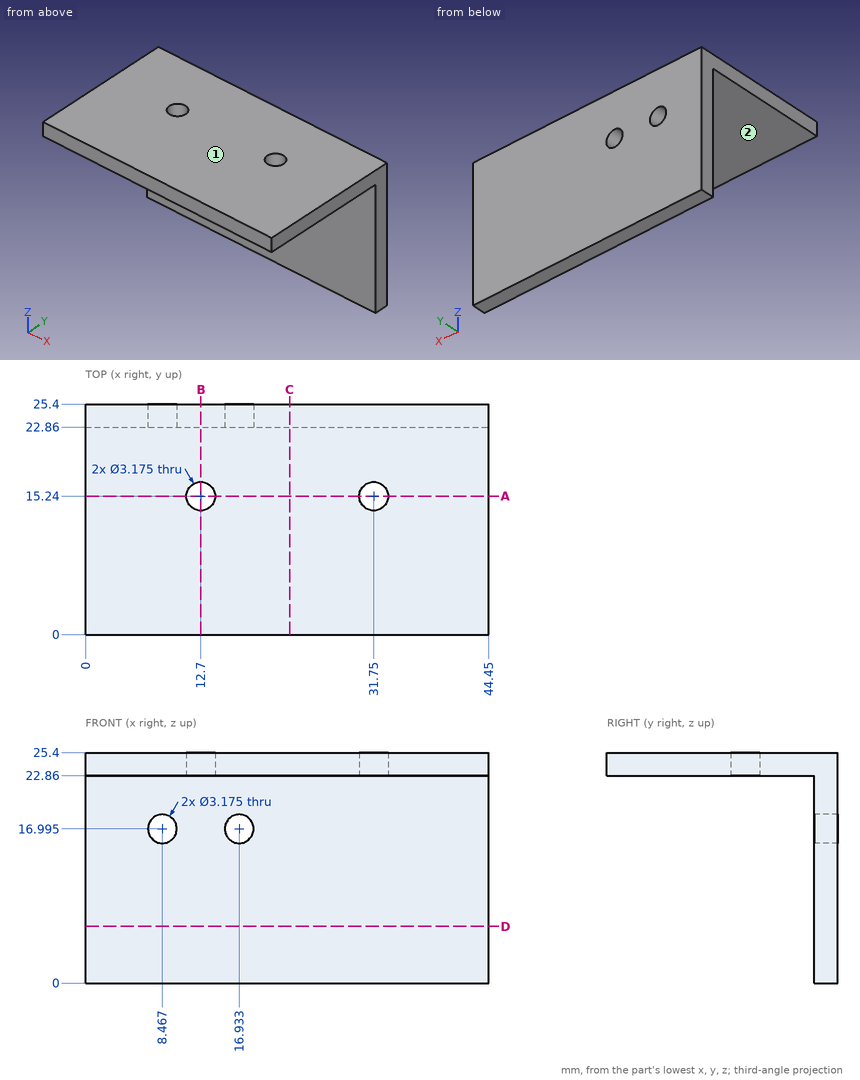
Geometry: see drawing. Coordinates: mm, zero at the bounding-box minimum. A direction names the side the tool comes from. Give positions to 0.01 mm unless a question says otherwise; leave off trailing zeros. Loops run counter-clockwise (first coordinate to the right, second up) from the corner with the lowest first, then second, coordinate; pieces in that order, holes last. Notation, with made-up numbers: (-31, 15) -> (15, 15) arc R4 ccw to (15, 21) -> close; hole circle Ø8 at (30, -16). An arc over 180 degrees is marked (long way). Answer as a JSON object with one key per item and string values. Group by question number.
Item 1: Line query: probe 1 along X at (y, z) = (24, 15.75); probe 2 along Y at (x, z) = (12.7, 24.6); probe 3 along Y at (x, z) = (26, 16.25). Output: solid intervals per line, ascending.
Item 2: Cut plane D-D, the plane z = 6.25. Return the cut outline in (x, y), and give its area (3 significant figures).
Item 3: Pin query (flat end, axial travel): P1, Ø4, axis at x = 8.47, z = 16.99, coming from the +Y side; P2, Ø4, axis at x = 27.5, y = 19, coming from the -Z side; P3, Ø3, axis at x = 35.5, z = 17, coming from the -Y side. Return the tip coordinate at first contact, or that it passes through.
Item 4: Reachability of the marked faces 1 and 2 from +Z, -Z, +X, -X, +Y, -Y: full face, straight path, thin tool, end or side. Return the list, or none.
Item 5: Cut plane B-B, the plane x = 12.7. Return the cut outline in (y, z).
Item 6: Cut plane A-A, the plane y = 15.24. Return the cut outline in (x, z).
Item 7: Cut plane C-C, the plane x = 22.5. Return the cut outline in (y, z).
Checks:
{
 "1": {"probe 1": "x = 0 to 7.48, 9.45 to 15.95, 17.92 to 44.45", "probe 2": "y = 0 to 13.65, 16.83 to 25.4", "probe 3": "y = 22.86 to 25.4"},
 "2": {"outline": "(0, 22.86) -> (44.45, 22.86) -> (44.45, 25.4) -> (0, 25.4) -> close", "area": "113 mm²"},
 "3": {"P1": "stops at y = 25.4", "P2": "stops at z = 22.86", "P3": "stops at y = 22.86"},
 "4": {"face 1": "+Z, +X, -X, +Y, -Y", "face 2": "-Z, +X, -X, -Y"},
 "5": {"outline": "(0, 22.86) -> (13.65, 22.86) -> (13.65, 25.4) -> (0, 25.4) -> close; (16.83, 22.86) -> (22.86, 22.86) -> (22.86, 0) -> (25.4, 0) -> (25.4, 25.4) -> (16.83, 25.4) -> close"},
 "6": {"outline": "(0, 22.86) -> (11.11, 22.86) -> (11.11, 25.4) -> (0, 25.4) -> close; (14.29, 22.86) -> (30.16, 22.86) -> (30.16, 25.4) -> (14.29, 25.4) -> close; (33.34, 22.86) -> (44.45, 22.86) -> (44.45, 25.4) -> (33.34, 25.4) -> close"},
 "7": {"outline": "(0, 22.86) -> (22.86, 22.86) -> (22.86, 0) -> (25.4, 0) -> (25.4, 25.4) -> (0, 25.4) -> close"}
}
